```python
from build123d import *

# Parameters (mm, degrees)
F1_DEPTH  = 32
F2_W      = 35
F2_H      = 17
F4_DEPTH  = 32
F5_DEPTH  = 25
F6_R      = 6.5
F7_DEPTH  = 80
F9_DEPTH  = 80
F11_DEPTH = 25
F13_DEPTH = 25


with BuildPart() as f1:
    # F0 (on Front) → F1 (new body)
    with BuildSketch(Plane.XZ):
        Polygon((0, 0), (39, 0), (74, 0), (113, 0), (113, 13), (88, 13), (88, 64), (69, 64), (69, 30), (44, 30), (44, 64), (25, 64), (25, 13), (0, 13), align=None)
    extrude(amount=-F1_DEPTH)

    # F2 (on face) → F4 (cut)
    with BuildSketch(Plane.XZ):
        with Locations((56.5, 8.5)):
            Rectangle(F2_W, F2_H)
    extrude(amount=-F4_DEPTH, mode=Mode.SUBTRACT)

    # F3 (on face) → F5 (cut)
    with BuildSketch(Plane.XY.offset(13)):
        with BuildLine():
            ThreePointArc((106.5, 19), (101, 24.5), (95.5, 19))
            ThreePointArc((95.5, 19), (101, 13.5), (106.5, 19))
        make_face()
        with BuildLine():
            ThreePointArc((7.5, 19), (13, 13.5), (18.5, 19))
            ThreePointArc((18.5, 19), (13, 24.5), (7.5, 19))
        make_face()
    extrude(amount=-F5_DEPTH, mode=Mode.SUBTRACT)

    # F6 (on face) → F7 (cut)
    with BuildSketch(Plane.YZ.offset(88)):
        with Locations((16, 46)):
            Circle(F6_R)
    extrude(amount=-F7_DEPTH, mode=Mode.SUBTRACT)

    # F8 (on face) → F9 (cut)
    with BuildSketch(Plane.YZ.offset(88)):
        with BuildLine():
            ThreePointArc((0, 60.4506665125), (16.1110103603, 63.8650900471), (32, 59.5334678182))
            Line((32, 59.5334678182), (32, 64))
            Line((32, 64), (0, 64))
            Line((0, 64), (0, 60.4506665125))
        make_face()
    extrude(amount=-F9_DEPTH, mode=Mode.SUBTRACT)

    # F10 (on face) → F11 (cut)
    with BuildSketch(Plane.XY.offset(13)):
        Polygon((104.471758008, 0), (113, 0), (113, 8.528241992), align=None)
    extrude(amount=-F11_DEPTH, mode=Mode.SUBTRACT)

    # F12 (on face) → F13 (cut)
    with BuildSketch(Plane.XY.offset(13)):
        Polygon((0, 12.873), (0, 0), (12.5, 0), align=None)
    extrude(amount=-F13_DEPTH, mode=Mode.SUBTRACT)


solid = f1.part
```
CAD build for the part. Positions are in the model's coordinates, mm. A direction names the side the tool comes from. Round coordinates to 2 decimals unless told otherwise and drop trailing zeros. Write each loop counter-clockwise with the first axis right and the second up, starting at its lowest first coordinate (ties: lowest second). Pieces come first, ordered by that corner, then holes. Notation, with made-up numbers: (50.5, -37.75) -> (56.5, -37.75) arc R16 cw to (56.5, -13.75) -> close; hole circle Ø1 at (-28, 25.25). An arc over 180 degrees is marked (long way). Answer in a Markdown table with one row per item. Add a question column.
Item 1: Saw through at B-B, the plane x = 101. Write the cut outline in (y, z), then the cut area to 3 significant figures.
Item 2: Which spindle directions (+Z, -Z, +X, -X, +Y, -Y) get a long thin tool onto all of the face, cutting with end or side? Do faces 1 (the face through (13, 12, 13)), 2 (the face through (39, 16, 8)), 3 (the face through (101, 12, 13)), 4 (the face through (93, 16, 0)), 5 (the face through (44, 16, 39)). Say none if no direction does.
Item 3: Saw through at A-A, the plane z = 5. Write the cut outline in (x, y), then the cut area to 3 significant figures.
Item 4: Saw through at C-C, the plane z = 37.5. Write the cut outline in (x, y).
Item 5: Saw through at D-D, the plane y = 16. Count the separate pieces of the cut face and the enclosed holes in it, then the cut area to 3 significant figures.
Item 6: Drop flat-ended pins along their axis: pin 1 Ø3 at (x, y) = (91, 7) entering from +Z; pin 2 Ø12 at (y, z) = (11.5, 24) entering from +X; pin 3 Ø10 at (x, y) = (87.5, 21.5) entering from +Z. Give the stop position or say it passes through.
Item 7: Mould opens along X. For faces 6 (the face through (57, 16, 30)), 7 (the face through (25, 16, 39)), 8 (the face through (106.495, 18.758, 6.591)), 9 (the face through (78.633, 10.842, 42.045)) say: pulls with the +X half, pulls with the -X half, needs draft (parallel to the pull), parting line crosses it, or undercut.
Item 8: Drill centre lines: line 1 (Z direction, x = 34.25, y = 16); line 2 (X direction, y = 25, z = 7.5); line 3 (X direction, y = 28, z = 52.5). Where is each one in solid material? Low to high. Write a range as from..to.
Findings below:
| question | item | result |
|---|---|---|
| 1 | outline | (0, 0) -> (13.5, 0) -> (13.5, 13) -> (0, 13) -> close; (24.5, 0) -> (32, 0) -> (32, 13) -> (24.5, 13) -> close |
| 1 | area | 273 mm^2 |
| 2 | face 1 | +Z, -X, +Y, -Y |
| 2 | face 2 | -Z, +Y, -Y |
| 2 | face 3 | +Z, +X, +Y, -Y |
| 2 | face 4 | -Z, +X, -X, +Y, -Y |
| 2 | face 5 | +Z, +Y, -Y |
| 3 | outline | (0, 12.87) -> (12.5, 0) -> (39, 0) -> (39, 32) -> (0, 32) -> close; (74, 0) -> (104.47, 0) -> (113, 8.53) -> (113, 32) -> (74, 32) -> close; hole circle Ø11 at (13, 19); hole circle Ø11 at (101, 19) |
| 3 | area | 2,190 mm^2 |
| 4 | outline | (25, 0) -> (44, 0) -> (44, 32) -> (25, 32) -> close; (69, 0) -> (88, 0) -> (88, 32) -> (69, 32) -> close |
| 5 | separate pieces | 5 |
| 5 | enclosed holes | 0 |
| 5 | area | 2,500 mm^2 |
| 6 | pin 1 | stops at z = 13 |
| 6 | pin 2 | stops at x = 88 |
| 6 | pin 3 | stops at z = 63.85 |
| 7 | face 6 | undercut |
| 7 | face 7 | pulls with the -X half |
| 7 | face 8 | undercut |
| 7 | face 9 | needs draft |
| 8 | line 1 | z = 0..39.5, 52.5..63.87 |
| 8 | line 2 | x = 0..39, 74..113 |
| 8 | line 3 | x = 25..44, 69..88 |
